Here's how the part is built. I have some questions about the finished solid (model axes, mm). Face numbers are marked on the shaded views. A direction names the side the tool comes from. Coordinates: 2 decimals unless noted, no trailing zeros. Write each loop counter-clockwise with the first axis right and the second up, starting at its lowest first coordinate (ties: lowest second). Pieces come first, ordered by that corner, then holes. Notation, with made-up numbers: M 52,15.25 L 111,15.25 A26 ccw 111,33.25 Z; hole C 41.25,-11 d8. An arc over 180 degrees is marked long. Use a Markdown table: item, result.
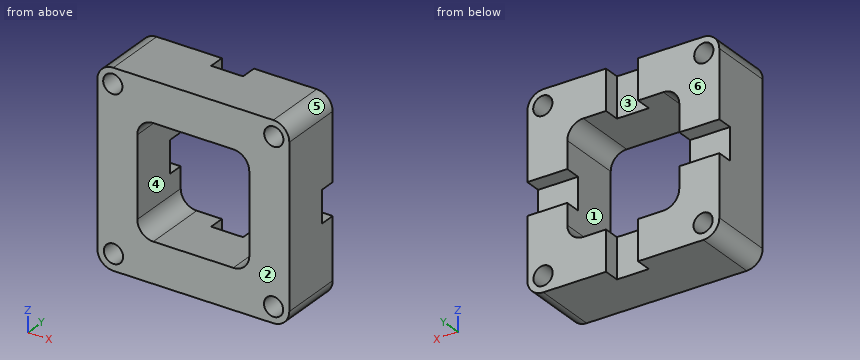
```python
from build123d import *

# Parameters (mm, degrees)
SKETCH1_R           = 6
SKETCH1_W           = 25
SKETCH1_H           = 20
SKETCH1_W_2         = 20
SKETCH1_H_2         = 25
BOSS_EXTRUDE1_DEPTH = 30
SKETCH2_R           = 6
BOSS_EXTRUDE2_DEPTH = 10


with BuildPart() as part:
    # Sketch1 → Boss-Extrude1 (new body)
    # profile 1 of 8: a face of its own
    with BuildSketch(Plane(origin=(0, 0, 0), x_dir=(1, 0, 0), z_dir=(0, 1, 0))):
        with BuildLine():
            Line((-9.676519666, -60), (-9.676519666, -35))
            Line((-9.676519666, -35), (-25, -35))
            ThreePointArc((-25, -35), (-32.071067812, -32.071067812), (-35, -25))
            Line((-35, -25), (-35, -7.678426698))
            Line((-35, -7.678426698), (-60, -7.678426698))
            Line((-60, -7.678426698), (-60, -50))
            ThreePointArc((-60, -50), (-57.071067812, -57.071067812), (-50, -60))
            Line((-50, -60), (-9.676519666, -60))
        make_face()
        with Locations(Location((-50.316110583, -50.316110583, 0), (0, 0, 270))):
            Circle(SKETCH1_R, mode=Mode.SUBTRACT)
    # profile 2 of 8: a face of its own
    with BuildSketch(Plane(origin=(0, 0, 0), x_dir=(1, 0, 0), z_dir=(0, 1, 0))):
        with BuildLine():
            Line((-60, 12.321573302), (-35, 12.321573302))
            Line((-35, 12.321573302), (-35, 25))
            ThreePointArc((-35, 25), (-32.071067812, 32.071067812), (-25, 35))
            Line((-25, 35), (-9.676519666, 35))
            Line((-9.676519666, 35), (-9.676519666, 60))
            Line((-9.676519666, 60), (-50, 60))
            ThreePointArc((-50, 60), (-57.071067812, 57.071067812), (-60, 50))
            Line((-60, 50), (-60, 12.321573302))
        make_face()
        with Locations(Location((-49.882833986, 49.882833986, 0), (0, 0, 270))):
            Circle(SKETCH1_R, mode=Mode.SUBTRACT)
    # profile 3 of 8: a face of its own
    with BuildSketch(Plane(origin=(0, 0, 0), x_dir=(1, 0, 0), z_dir=(0, 1, 0))):
        with BuildLine():
            Line((35, 25), (35, 12.321573302))
            Line((35, 12.321573302), (60, 12.321573302))
            Line((60, 12.321573302), (60, 50))
            ThreePointArc((60, 50), (57.071067812, 57.071067812), (50, 60))
            Line((50, 60), (10.323480334, 60))
            Line((10.323480334, 60), (10.323480334, 35))
            Line((10.323480334, 35), (25, 35))
            ThreePointArc((25, 35), (32.071067812, 32.071067812), (35, 25))
        make_face()
        with Locations(Location((50.17168505, 50.17168505, 0), (0, 0, 270))):
            Circle(SKETCH1_R, mode=Mode.SUBTRACT)
    # profile 4 of 8: a face of its own
    with BuildSketch(Plane(origin=(0, 0, 0), x_dir=(1, 0, 0), z_dir=(0, 1, 0))):
        with BuildLine():
            Line((25, -35), (10.323480334, -35))
            Line((10.323480334, -35), (10.323480334, -60))
            Line((10.323480334, -60), (50, -60))
            ThreePointArc((50, -60), (57.071067812, -57.071067812), (60, -50))
            Line((60, -50), (60, -7.678426698))
            Line((60, -7.678426698), (35, -7.678426698))
            Line((35, -7.678426698), (35, -25))
            ThreePointArc((35, -25), (32.071067812, -32.071067812), (25, -35))
        make_face()
        with Locations(Location((50.316110583, -50.316110583, 0), (0, 0, 270))):
            Circle(SKETCH1_R, mode=Mode.SUBTRACT)
    # profile 5 of 8: a face of its own
    with BuildSketch(Plane(origin=(0, 0, 0), x_dir=(1, 0, 0), z_dir=(0, 1, 0))):
        with Locations((-47.5, 2.321573302)):
            Rectangle(SKETCH1_W, SKETCH1_H)
    # profile 6 of 8: a face of its own
    with BuildSketch(Plane(origin=(0, 0, 0), x_dir=(1, 0, 0), z_dir=(0, 1, 0))):
        with Locations((47.5, 2.321573302)):
            Rectangle(SKETCH1_W, SKETCH1_H)
    # profile 7 of 8: a face of its own
    with BuildSketch(Plane(origin=(0, 0, 0), x_dir=(1, 0, 0), z_dir=(0, 1, 0))):
        with Locations((0.323480334, 47.5)):
            Rectangle(SKETCH1_W_2, SKETCH1_H_2)
    # profile 8 of 8: a face of its own
    with BuildSketch(Plane(origin=(0, 0, 0), x_dir=(1, 0, 0), z_dir=(0, 1, 0))):
        with Locations((0.323480334, -47.5)):
            Rectangle(SKETCH1_W_2, SKETCH1_H_2)
    extrude(amount=BOSS_EXTRUDE1_DEPTH)

    # Sketch2 → Boss-Extrude2 (add)
    # profile 1 of 4: a face of its own
    with BuildSketch(Plane(origin=(0, 30, 0), x_dir=(1, 0, 0), z_dir=(0, 1, 0))):
        with BuildLine():
            Line((-9.228273843, 35), (-9.228273843, 60))
            Line((-9.228273843, 60), (-50, 60))
            ThreePointArc((-50, 60), (-57.071067812, 57.071067812), (-60, 50))
            Line((-60, 50), (-60, 11.816725799))
            Line((-60, 11.816725799), (-35, 11.816725799))
            Line((-35, 11.816725799), (-35, 25))
            ThreePointArc((-35, 25), (-32.071067812, 32.071067812), (-25, 35))
            Line((-25, 35), (-9.228273843, 35))
        make_face()
        with Locations(Location((-49.882833986, 49.882833986, 0), (0, 0, 270))):
            Circle(SKETCH2_R, mode=Mode.SUBTRACT)
    # profile 2 of 4: a face of its own
    with BuildSketch(Plane(origin=(0, 30, 0), x_dir=(1, 0, 0), z_dir=(0, 1, 0))):
        with BuildLine():
            Line((50, 60), (10.771726157, 60))
            Line((10.771726157, 60), (10.771726157, 35))
            Line((10.771726157, 35), (25, 35))
            ThreePointArc((25, 35), (32.071067812, 32.071067812), (35, 25))
            Line((35, 25), (35, 11.816725799))
            Line((35, 11.816725799), (60, 11.816725799))
            Line((60, 11.816725799), (60, 50))
            ThreePointArc((60, 50), (57.071067812, 57.071067812), (50, 60))
        make_face()
        with Locations(Location((50.17168505, 50.17168505, 0), (0, 0, 270))):
            Circle(SKETCH2_R, mode=Mode.SUBTRACT)
    # profile 3 of 4: a face of its own
    with BuildSketch(Plane(origin=(0, 30, 0), x_dir=(1, 0, 0), z_dir=(0, 1, 0))):
        with BuildLine():
            Line((60, -50), (60, -8.183274201))
            Line((60, -8.183274201), (35, -8.183274201))
            Line((35, -8.183274201), (35, -25))
            ThreePointArc((35, -25), (32.071067812, -32.071067812), (25, -35))
            Line((25, -35), (10.771726157, -35))
            Line((10.771726157, -35), (10.771726157, -60))
            Line((10.771726157, -60), (50, -60))
            ThreePointArc((50, -60), (57.071067812, -57.071067812), (60, -50))
        make_face()
        with Locations(Location((50.316110583, -50.316110583, 0), (0, 0, 270))):
            Circle(SKETCH2_R, mode=Mode.SUBTRACT)
    # profile 4 of 4: a face of its own
    with BuildSketch(Plane(origin=(0, 30, 0), x_dir=(1, 0, 0), z_dir=(0, 1, 0))):
        with BuildLine():
            Line((-35, -8.183274201), (-60, -8.183274201))
            Line((-60, -8.183274201), (-60, -50))
            ThreePointArc((-60, -50), (-57.071067812, -57.071067812), (-50, -60))
            Line((-50, -60), (-9.228273843, -60))
            Line((-9.228273843, -60), (-9.228273843, -35))
            Line((-9.228273843, -35), (-25, -35))
            ThreePointArc((-25, -35), (-32.071067812, -32.071067812), (-35, -25))
            Line((-35, -25), (-35, -8.183274201))
        make_face()
        with Locations(Location((-50.316110583, -50.316110583, 0), (0, 0, 270))):
            Circle(SKETCH2_R, mode=Mode.SUBTRACT)
    extrude(amount=BOSS_EXTRUDE2_DEPTH)


solid = part.part
```
1. I need wall thicknesses on probe 1 along Z at (x, y) = (2.5, 9); probe 2 along Z at (x, y) = (-42.5, 32.5). Which ranges of each line are inside material? Lowest first, please.
Answers follow:
| item | result |
|---|---|
| probe 1 | z = -60 to -35, 35 to 60 |
| probe 2 | z = -60 to -11.82, 8.18 to 60 |
2. Suppose I cut it at D-D on x = -39. Write out the boundary of the cut face in (y, z), and give its area (3 significant figures).
Answers follow:
| item | result |
|---|---|
| outline | M 0,-60 L 40,-60 L 40,-11.82 L 30,-11.82 L 30,8.18 L 40,8.18 L 40,60 L 0,60 Z |
| area | 4,600 mm2 |
3. Which directions (+Z, -Z, +X, -X, +Y, -Y) give clear straight access to the entire face, cutting with the end or side of a thin tool? Please do the marked faces 1, 2 and 3.
Answers follow:
| item | result |
|---|---|
| face 1 | +Y, -Y |
| face 2 | +Z, -Z, +X, -X, -Y |
| face 3 | +Z, -Z, +Y |
4. Suppose I cut it at B-B on z = 6. Write out the boundary of the cut face in (x, y), and give its area (3 significant figures).
Answers follow:
| item | result |
|---|---|
| outline | M -60,0 L -35,0 L -35,30 L -60,30 Z; M 35,0 L 60,0 L 60,30 L 35,30 Z |
| area | 1,500 mm2 |
5. We'd pull the mould along Z, two halves only. Please class the marked faces 4, 5 and 6: +Z half, -Z half, draft (parallel to the pull), parting line (faces both ways), or undercut.
Answers follow:
| item | result |
|---|---|
| face 4 | undercut |
| face 5 | +Z half |
| face 6 | draft |
6. Suppose I cut it at A-A on x = 22.5. Write out the boundary of the cut face in (y, z), and give its area (3 significant figures).
Answers follow:
| item | result |
|---|---|
| outline | M 0,-60 L 40,-60 L 40,-35 L 0,-35 Z; M 0,35 L 40,35 L 40,60 L 0,60 Z |
| area | 2,000 mm2 |
7. Will these pins go through, and if not, where does the flat tip stop? pin 1 Ø16 at (x, z) = (6, 49.5) entering from +Y; pin 2 Ø9.5 at (x, z) = (-50.32, 50.32) entering from +Y.
Answers follow:
| item | result |
|---|---|
| pin 1 | stops at y = 40 |
| pin 2 | passes through |
8. Suppose I cut it at C-C on z = -38.5. Write out the boundary of the cut face in (x, y).
Answers follow:
| item | result |
|---|---|
| outline | M -60,0 L 60,0 L 60,40 L 10.77,40 L 10.77,30 L -9.23,30 L -9.23,40 L -60,40 Z |
